Verification items for this drawing (mm, ordinates from the low corner). Coordinates: 2 decimals unless noted, no trailing zeros. Order: outer loops, then holes, each group sorted by start corner. A loop starts at its lowest first (then second) coordinate and runs counter-clockwise, first axis right, second up. Notation, with made-up numbers: (29.5, -29) -> (61.5, -29) arc R34 ccw to (61.5, 8) -> close; hole circle Ø4 at (-13, -4.5). An arc over 180 degrees is marked (long way). Write each question's results on one line, items separated by ' | '. Start each with the question number.
(1) Cross-section at B-B on x = 44. Enter the section's corners in (y, z).
(2) Cross-section at A-A on y = 0.65. Enter the section's corners in (x, z), and give its area (3 significant figures).
(3) Thickness scan on probe 1 along Z at (x, y) = (15, 0.75); probe 2 along Z at (x, y) = (54, 0.3); probe 3 along X at (y, z) = (0.8, 12) (1 decimal). Record the ranges inside material, lowest first. Write a range as [from, to].
(4) Cross-section at C-C on z = 8. Enter the section's corners in (x, y), and give its area (3 significant figures).
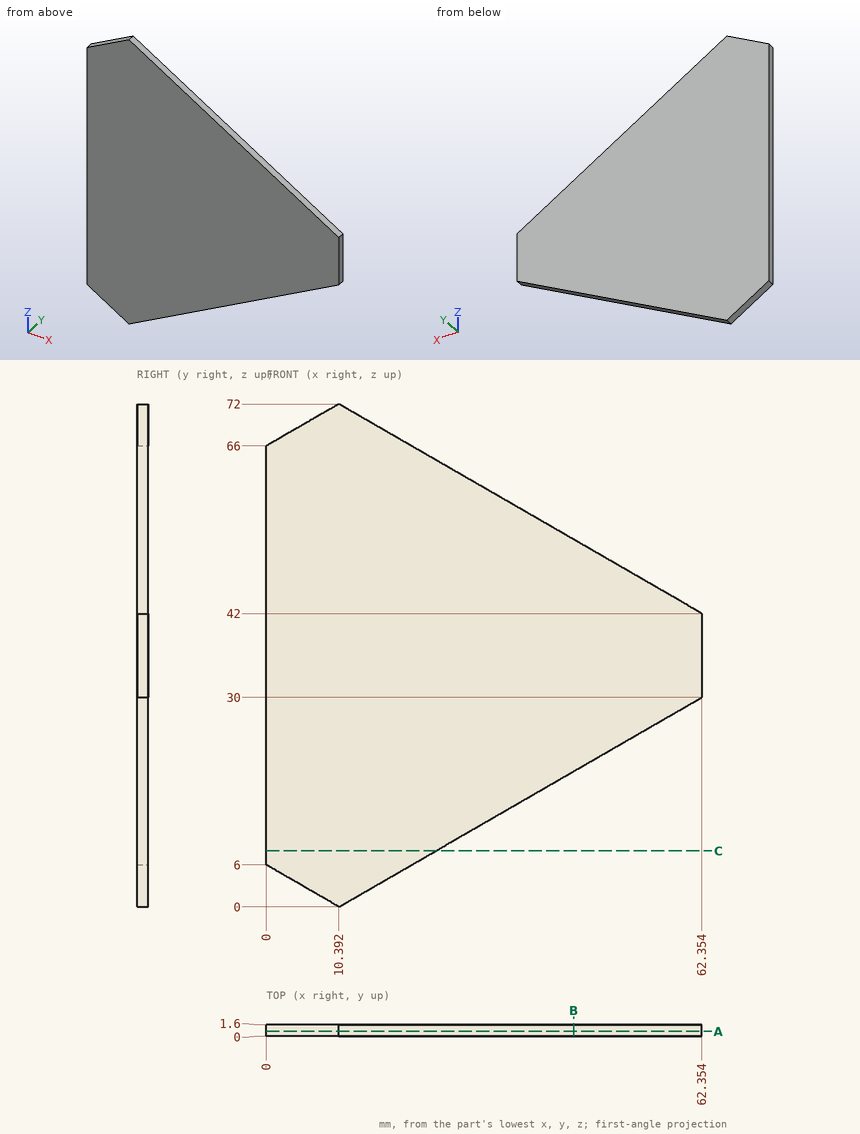
Results are:
1) outline: (0, 19.4) -> (1.6, 19.4) -> (1.6, 52.6) -> (0, 52.6) -> close
2) outline: (0, 6) -> (10.39, 0) -> (62.35, 30) -> (62.35, 42) -> (10.39, 72) -> (0, 66) -> close | area: 2,870 mm2
3) probe 1: z = [2.66, 69.34] | probe 2: z = [25.18, 46.82] | probe 3: x = [0, 31.2]
4) outline: (0, 0) -> (24.25, 0) -> (24.25, 1.6) -> (0, 1.6) -> close | area: 38.8 mm2
